Design review of the part built by this model. Coordinates are the model's own, in mm. A direction names the side the tool comes from. Round coordinates to 2 decimals unless told otherwise and drop trailing zeros. Loops run counter-clockwise (first coordinate to the right, second up) from the corner with the lowest first, then second, coordinate; pieces in that order, holes last. Notation, with made-up numbers: (32.5, -30) -> (61.5, -30) arc R22 ccw to (61.5, 3) -> close; hole circle Ø10 at (-20, 27.25). An arc over 180 degrees is marked (long way). Answer as CSV lines item,"result". Start each with the question number.
(1) Take a section at A-A, the plane z = 14.5. Write out the cut boundary in (x, y).
(2) Take a section at B-B, the plane x = -9.5. Write out the cut boundary in (y, z), and give its area (3 significant figures).
(3) Take a section at C-C, the plane y = -14.5. Write out the cut boundary in (x, z).
(4) Draft analysis for pull direction X (two halves, no side actions). For faces 6 (the face through (6, 0, 11)), 7 (the face through (0, 12, 23)), 8 (the face through (6.5, 0, 12)), 9 (the face through (-0.217, -15.476, 22.507)), state which applies: +X half, -X half, draft (parallel to the pull), parting line (faces both ways), or undercut.
(5) Take a section at D-D, the plane y = -2. Write out the cut boundary in (x, z), and give its area (3 significant figures).
(6) To check wall thickness, follow line 1 (X direction, y = 0, z = 5); line 2 (Y direction, x = 0, z = 22.85); line 3 (Y direction, x = 4.5, z = 12.25). State the ranges of each line that lie inside material, in increasing order. Write a range as from..to.
(7) Machinability: for faces 1 (the face through (-0.1, 17, 22.5)), 2 (the face through (-15.85, 3, 11.03)), 3 (the face through (-7, -3.75, 11)), 4 (the face through (0, -13, 22)), 5 (the face through (0, 16, 22)), which of the approach directions +Z, -Z, +X, -X, +Y, -Y give a long, thin tool a straight path to every point of the face, cutting with its end or side? Answer none if there is none.
(8) For P1, Ø3, axis at x = 1.5, y = 15.5, coming from the -Z side; P2, Ø5, axis at x = -9.5, z = 10, coming from the -Y side; P3, Ø4, axis at x = 2.5, z = 9.5, coming from the -Y side, all flat-tipped, find the tip position at first contact; note any pin that passes through.
from build123d import *

# Parameters (mm, degrees)
SKETCH1_W           = 13
SKETCH1_H           = 23
BOSS_EXTRUDE1_DEPTH = 23
CUT_EXTRUDE1_REACH  = 25
SKETCH1_3_W         = 12
SKETCH1_3_H         = 22
SKETCH2_W           = 13
SKETCH2_H           = 5.5
SKETCH2_R           = 1
BOSS_EXTRUDE2_DEPTH = 1
SKETCH4_W           = 13
SKETCH4_H           = 7.5
BOSS_EXTRUDE3_DEPTH = 10
CUT_EXTRUDE2_REACH  = 22.75
SKETCH5_W           = 8
SKETCH5_H           = 11
CUT_EXTRUDE3_REACH  = 19.5
SKETCH6_W           = 9
SKETCH6_H           = 6


with BuildPart() as part:
    # Sketch1 → Boss-Extrude1 (new body)
    with BuildSketch(Plane.XY):
        Rectangle(SKETCH1_W, SKETCH1_H)
    extrude(amount=BOSS_EXTRUDE1_DEPTH)

    # Sketch1_3 → Cut-Extrude1 (cut, up to next)
    with BuildSketch(Plane.XY, mode=Mode.PRIVATE) as cut_extrude1_sk1:
        Rectangle(SKETCH1_3_W, SKETCH1_3_H)
    cut_extrude1_tool1 = extrude(cut_extrude1_sk1.sketch, amount=CUT_EXTRUDE1_REACH, mode=Mode.PRIVATE) & part.part
    add(cut_extrude1_tool1.solids().sort_by_distance((0, 0, 0))[0], mode=Mode.SUBTRACT)

    # Sketch2 → Boss-Extrude2 (add)
    with BuildSketch(Plane.XY.offset(23)):
        with Locations((0, 14.25)):
            Rectangle(SKETCH2_W, SKETCH2_H)
        with Locations((0, 14.5)):
            Circle(SKETCH2_R, mode=Mode.SUBTRACT)
        with Locations((0, -14.25)):
            Rectangle(SKETCH2_W, SKETCH2_H)
        with Locations((0, -14.5)):
            Circle(SKETCH2_R, mode=Mode.SUBTRACT)
    extrude(amount=-BOSS_EXTRUDE2_DEPTH)

    # Sketch4 → Boss-Extrude3 (add)
    with BuildSketch(Plane.ZY.offset(6.5)):
        with Locations((11, 0)):
            Rectangle(SKETCH4_W, SKETCH4_H)
    extrude(amount=BOSS_EXTRUDE3_DEPTH)

    # Sketch5 → Cut-Extrude2 (cut, up to next)
    with BuildSketch(Plane(origin=(0, -3.75, 0), x_dir=(-1, 0, 0), z_dir=(0, -1, 0)), mode=Mode.PRIVATE) as cut_extrude2_sk1:
        with Locations((11.5, -11)):
            Rectangle(SKETCH5_W, SKETCH5_H)
    cut_extrude2_tool1 = extrude(cut_extrude2_sk1.sketch, amount=-CUT_EXTRUDE2_REACH, mode=Mode.PRIVATE) & part.part
    add(cut_extrude2_tool1.solids().sort_by_distance((-11.5, -3.75, 11))[0], mode=Mode.SUBTRACT)

    # Sketch6 → Cut-Extrude3 (cut, up to next)
    with BuildSketch(Plane.XY.offset(17.5), mode=Mode.PRIVATE) as cut_extrude3_sk1:
        with Locations((-11.5, 0)):
            Rectangle(SKETCH6_W, SKETCH6_H)
    cut_extrude3_tool1 = extrude(cut_extrude3_sk1.sketch, amount=-CUT_EXTRUDE3_REACH, mode=Mode.PRIVATE) & part.part
    add(cut_extrude3_tool1.solids().sort_by_distance((-11.5, 0, 17.5))[0], mode=Mode.SUBTRACT)


solid = part.part
The answers:
1,outline,"(-16.5, -3.75) -> (-15.5, -3.75) -> (-15.5, -3) -> (-16, -3) -> (-16, 3) -> (-15.5, 3) -> (-15.5, 3.75) -> (-16.5, 3.75) -> close; (-7.5, -3.75) -> (-6.5, -3.75) -> (-6.5, -11.5) -> (6.5, -11.5) -> (6.5, 11.5) -> (-6.5, 11.5) -> (-6.5, 3.75) -> (-7.5, 3.75) -> (-7.5, 3) -> (-7, 3) -> (-7, -3) -> (-7.5, -3) -> close; hole (-6, -11) -> (6, -11) -> (6, 11) -> (-6, 11) -> close"
2,outline,"(-3.75, 4.5) -> (-3, 4.5) -> (-3, 5.5) -> (-3.75, 5.5) -> close; (-3.75, 16.5) -> (-3, 16.5) -> (-3, 17.5) -> (-3.75, 17.5) -> close; (3, 4.5) -> (3.75, 4.5) -> (3.75, 5.5) -> (3, 5.5) -> close; (3, 16.5) -> (3.75, 16.5) -> (3.75, 17.5) -> (3, 17.5) -> close"
2,area,"3.00 mm²"
3,outline,"(-6.5, 22) -> (-1, 22) -> (-1, 23) -> (-6.5, 23) -> close; (1, 22) -> (6.5, 22) -> (6.5, 23) -> (1, 23) -> close"
4,face 6,"undercut"
4,face 7,"draft"
4,face 8,"+X half"
4,face 9,"undercut"
5,outline,"(-16.5, 4.5) -> (-16, 4.5) -> (-16, 17.5) -> (-16.5, 17.5) -> close; (-7, 4.5) -> (-6.5, 4.5) -> (-6.5, 0) -> (-6, 0) -> (-6, 23) -> (-6.5, 23) -> (-6.5, 17.5) -> (-7, 17.5) -> close; (6, 0) -> (6.5, 0) -> (6.5, 23) -> (6, 23) -> close"
5,area,"36.0 mm²"
6,line 1,"-16.5..-16, -7..-6, 6..6.5"
6,line 2,"-17..-15.5, -13.5..-11, 11..13.5, 15.5..17"
6,line 3,"-11.5..-11, 11..11.5"
7,face 1,"+Z, -Z, +X, -X, +Y"
7,face 2,"+Z, -Z"
7,face 3,"+Z, -Z, -X, -Y"
7,face 4,"-Z, +X, -X, -Y"
7,face 5,"-Z, +X, -X, +Y"
8,P1,"z = 22"
8,P2,"y = -3.75"
8,P3,"y = -11.5"
